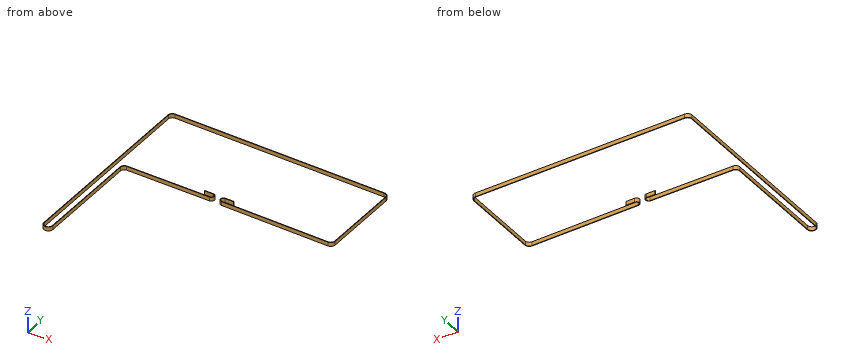
Autodesk Inventor part; units mm, degrees
ref_plane "Work Plane2" through (168.6815, -122.8197, 0) normal (0.9993154, -0.0369972, 0) x (0.0369972, 0.9993154, 0)
ref_plane "YZ Plane" through (0, 0, 0) normal (1, 0, 0) x (0, 1, 0)
ref_plane "XZ Plane" through (0, 0, 0) normal (0, 1, 0) x (-1, 0, 0)
sketch "Sketch1" plane through (0, 0, 0) normal (0, 0, 1) x (1, 0, 0)
  circle A0 centre (0, 0) radius 6.05
surface extrude "ExtrusionSrf1" sketch "Sketch1" along normal mid plane 6 shown yes curves A0
sketch "Sketch2" plane through (0, 0, 0) normal (0, 0, 1) x (1, 0, 0)
  circle A0 centre (324.834, -10.3853) radius 6.05
  point P0 (0, 0)
surface extrude "ExtrusionSrf2" sketch "Sketch2" along normal mid plane 6 shown yes curves A0
sketch "Sketch3" plane through (0, 0, 0) normal (0, 0, 1) x (1, 0, 0)
  circle A0 centre (-9.3308, -291.8509) radius 6.11
  point P0 (0, 0)
surface extrude "ExtrusionSrf3" sketch "Sketch3" along normal blind 6 shown yes curves A0
sketch "Sketch4" plane through (0, 0, 0) normal (0, 0, 1) x (1, 0, 0)
  circle A0 centre (8.4872, -132.9103) radius 5.735
  point P0 (0, 0)
surface extrude "ExtrusionSrf4" sketch "Sketch4" along normal mid plane 6 shown yes curves A0
sketch "Sketch5" plane through (0, 0, 0) normal (0, 0, 1) x (1, 0, 0)
  circle A0 centre (321.0045, -130.1653) radius 6.05
  point P0 (0, 0)
surface extrude "ExtrusionSrf5" sketch "Sketch5" along normal mid plane 6 shown yes curves A0
sketch "Sketch6" plane through (0, 0, 0) normal (0, 0, 1) x (1, 0, 0)
  circle A0 centre (136.5519, -125.7339) radius 3
  point P0 (0, 0)
surface extrude "ExtrusionSrf6" sketch "Sketch6" along normal mid plane 6 shown yes curves A0
sketch "Sketch7" plane through (0, 0, 0) normal (0, 0, 1) x (1, 0, 0)
  circle A0 centre (155.5422, -126.341) radius 3
  point P0 (0, 0)
surface extrude "ExtrusionSrf7" sketch "Sketch7" along normal mid plane 6 shown yes curves A0
sketch "Sketch8" plane through (0, 0, 0) normal (0, 0, 1) x (1, 0, 0)
  circle A0 centre (0, 0) radius 6.05
  circle A1 centre (8.4872, -132.9103) radius 5.735
  circle A2 centre (-9.3308, -291.8509) radius 6.11
  circle A3 centre (136.5519, -125.7339) radius 3
  circle A4 centre (155.5422, -126.341) radius 3
  circle A5 centre (321.0045, -130.1653) radius 6.05
  circle A6 centre (324.834, -10.3853) radius 6.05
  arc A7 (0.2015, 6.3018) -> (-6.3017, 0.2028) centre (0, 0) ccw
  arc A8 (-15.6925, -291.6462) -> (-2.969, -292.0543) centre (-9.3308, -291.8509) ccw
  arc A9 (8.6461, -126.5472) -> (2.1255, -132.7069) centre (8.4872, -132.9103) ccw
  arc A10 (136.452, -129.7376) -> (136.6519, -121.7301) centre (136.5519, -125.7339) ccw
  arc A11 (331.1358, -10.5868) -> (325.0355, -4.0835) centre (324.834, -10.3853) ccw
  arc A12 (155.6904, -122.3388) -> (155.3941, -130.3433) centre (155.5422, -126.341) ccw
  arc A13 (320.7713, -136.466) -> (327.3063, -130.3668) centre (321.0045, -130.1653) ccw
  line L0 (-15.6925, -291.6462) -> (-6.3017, 0.2028)
  line L1 (0.2015, 6.3018) -> (325.0355, -4.0835)
  line L2 (-2.969, -292.0543) -> (2.1255, -132.7069)
  line L3 (8.6461, -126.5472) -> (136.452, -129.7376)
  line L4 (331.1358, -10.5868) -> (327.3063, -130.3668)
  line L5 (123.6519, -121.4056) -> (136.6519, -121.7301)
  line L6 (155.3941, -130.3433) -> (320.7713, -136.466)
  line L7 (155.6904, -122.3388) -> (168.6815, -122.8197)
  dimension "d14" = 0.255
  dimension "d15" = 0.255
  dimension "d16" = 0.255
  dimension "d17" = 0.63
  dimension "d19" = 0.255
  dimension "d22" = 1.005
  dimension "d23" = 1.005
  dimension "d34" = 13
  dimension "d35" = 13
ref_plane "Work Plane2" through (168.6815, -122.8197, 0) normal (0.9993154, -0.0369972, 0) x (0.0369972, 0.9993154, 0)
sketch "Sketch10" plane through (168.6815, -122.8197, 0) normal (0.9993154, -0.0369972, 0) x (0.0369972, 0.9993154, 0)
  line L0 (0.63, 3) -> (-0.255, 3)
  line L1 (-0.255, 3) -> (-0.255, -3)
  line L2 (-0.255, -3) -> (0.63, -3)
  line L3 (0.63, -3) -> (0.63, 3)
  line L4 (0.63, 0) -> (-0.255, 0) construction
  point P0 (116.4949, 0)
  point P1 (0, 0)
  dimension "d29" = 6
  dimension "d30" = 0.63
  dimension "d31" = 0.255
sweep "Sweep2" add profiles "Sketch10" path "Sketch8" path curves L7 A12 L6 A13 L4 A11 L1 A7 L0 A8 L2 A9 L3 A10 L5
equation "\"d14\" = inside"
equation "\"d15\" = inside"
equation "\"d16\" = inside"
equation "\"d17\" = backside"
equation "\"d19\" = inside"
equation "\"inside\" = 0.255"
equation "\"backside\" = 0.63"
properties part number "Belt 3" material "Rubber"
Input: part model. Units: mm. Frame: model coordinates. Give positions to 0.01 mm unless a question says otherwise; leave off trailing zeros. Order: outer loops, then holes, each group sorted by start corner. A loop starts at its lowest first (then second) coordinate and runs counter-clockwise, first axis right, second up. Notation, with made-up numbers: M 29,76.5 L 85,76.5 A23 cw 85,114.5 Z; hole C 78,51 d4. An arc over 180 degrees is marked long. Answer as a JSON object with one key per item and string values.
1. Cut plane B-B, the plane x = 277. Output: boundary loops of the cut face in (y, z).
Result sheet:
{"outline": "M -135.48,-3 L -134.59,-3 L -134.59,3 L -135.48,3 Z; M -2.8,-3 L -1.92,-3 L -1.92,3 L -2.8,3 Z"}
2. First-contact query: P1, Ø1.5, axis at x = 160, z = 1, coming from the -Y side; P2, Ø2, axis at x = 128.5, z = 0, coming from the +Y side; P3, Ø1.5, axis at x = 70.5, z = -0.5, coming from the +Y side. Flat tips, straight axial feed; report the tip coordinate or a pass-through.
Result sheet:
{"P1": "y = -131.17", "P2": "y = 2.86", "P3": "y = 4.71"}
3. Ray query, line 1 (Y direction, x = 157.5, z = 0.75); line 2 (Y direction, x = 154, z = 2.7); line 3 (X direction, y = -43, z = 0.95). Return the intervals inside material, ascending. Write a range as [from, to].
Result sheet:
{"line 1": "[-131.05, -130.17], [-122.66, -121.78], [1.02, 1.9]", "line 2": "[-130.71, -129.76], [-122.92, -121.97], [1.13, 2.02]", "line 3": "[-8.32, -7.44], [329.84, 330.73]"}
4. Cut plane A-A, the plane y = -66. Output: boundary loops of the cut face in (x, z), and give its area (3 significant figures).
Result sheet:
{"outline": "M -9.06,-3 L -8.18,-3 L -8.18,3 L -9.06,3 Z; M 329.11,-3 L 329.99,-3 L 329.99,3 L 329.11,3 Z", "area": "10.6 mm²"}
